```python
from build123d import *

# Parameters (mm, degrees)
BOSS_EXTRUDE1_DEPTH = 1.5


with BuildPart() as part:
    # Sketch1 → Boss-Extrude1 (new, symmetric)
    with BuildSketch(Plane(origin=(0, 0, 0), x_dir=(1, 0, 0), z_dir=(0, 1, 0))):
        Polygon((49.5, 50), (40.5, 50), (40.5, 47), (31.5, 47), (31.5, 50), (22.5, 50), (22.5, 47), (13.5, 47), (13.5, 50), (4.5, 50), (4.5, 47), (-4.5, 47), (-4.5, 50), (-13.5, 50), (-13.5, 47), (-22.5, 47), (-22.5, 50), (-31.5, 50), (-31.5, 47), (-40.5, 47), (-40.5, 50), (-49.5, 50), (-49.5, 47), (-54, 47), (-54, 40.5), (-57, 40.5), (-57, 31.5), (-54, 31.5), (-54, 22.5), (-57, 22.5), (-57, 13.5), (-54, 13.5), (-54, 4.5), (-57, 4.5), (-57, -4.5), (-54, -4.5), (-54, -13.5), (-57, -13.5), (-57, -22.5), (-54, -22.5), (-54, -31.5), (-57, -31.5), (-57, -40.5), (-54, -40.5), (-54, -47), (-49.5, -47), (-49.5, -50), (-40.5, -50), (-40.5, -47), (-31.5, -47), (-31.5, -50), (-22.5, -50), (-22.5, -47), (-13.5, -47), (-13.5, -50), (-4.5, -50), (-4.5, -47), (4.5, -47), (4.5, -50), (13.5, -50), (13.5, -47), (22.5, -47), (22.5, -50), (31.5, -50), (31.5, -47), (40.5, -47), (40.5, -50), (49.5, -50), (49.5, -47), (54, -47), (54, -40.5), (57, -40.5), (57, -31.5), (54, -31.5), (54, -22.5), (57, -22.5), (57, -13.5), (54, -13.5), (54, -4.5), (57, -4.5), (57, 4.5), (54, 4.5), (54, 13.5), (57, 13.5), (57, 22.5), (54, 22.5), (54, 31.5), (57, 31.5), (57, 40.5), (54, 40.5), (54, 47), (49.5, 47), align=None)
    extrude(amount=BOSS_EXTRUDE1_DEPTH, both=True)


solid = part.part
```
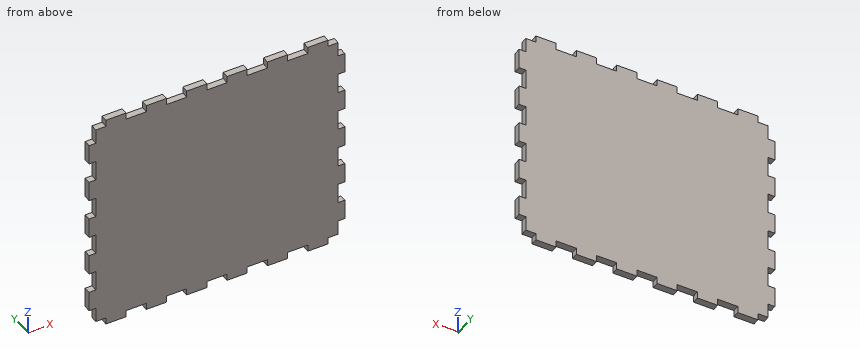
Work out the finished part from the listing and answer in its coordinate system (mm). Round coordinates to 2 decimals unless told otherwise and drop trailing zeros. Order: outer loops, then holes, each group sorted by start corner. A loop starts at its lowest first (then second) coordinate and runs counter-clockwise, first axis right, second up.
Q1. Given pin 1 Ø1.5 at (y, z) = (0, 44.5) entering from -X; pin 2 Ø1.5 at (x, y) = (-56, 0.5) entering from +Z; pin 3 Ø1.5 at (y, z) = (0, 48.5) entering from -X, each flat-ended and moving along its own axis, determine where each tip first touches the part or whether it passes through.
Solution:
pin 1: stops at x = -54
pin 2: stops at z = 40.5
pin 3: stops at x = -49.5
Q2. A cutting plane is placed at A-A, the plane x = 19. Determine the outline of the cut face in (y, z).
Solution:
outline: (-1.5, -47) - (1.5, -47) - (1.5, 47) - (-1.5, 47) - close
Q3. A cutting plane is placed at B-B, the plane z = 10.5. Determine the outline of the cut face in (x, y).
Solution:
outline: (-54, -1.5) - (54, -1.5) - (54, 1.5) - (-54, 1.5) - close
Q4. Find the intervals of material crossed by line 1 along X through (y, z) = (-0.9, -44.5); line 2 along Z through (x, y) = (16, -0.75), in increasing order.
Solution:
line 1: x = -54 to 54
line 2: z = -47 to 47
